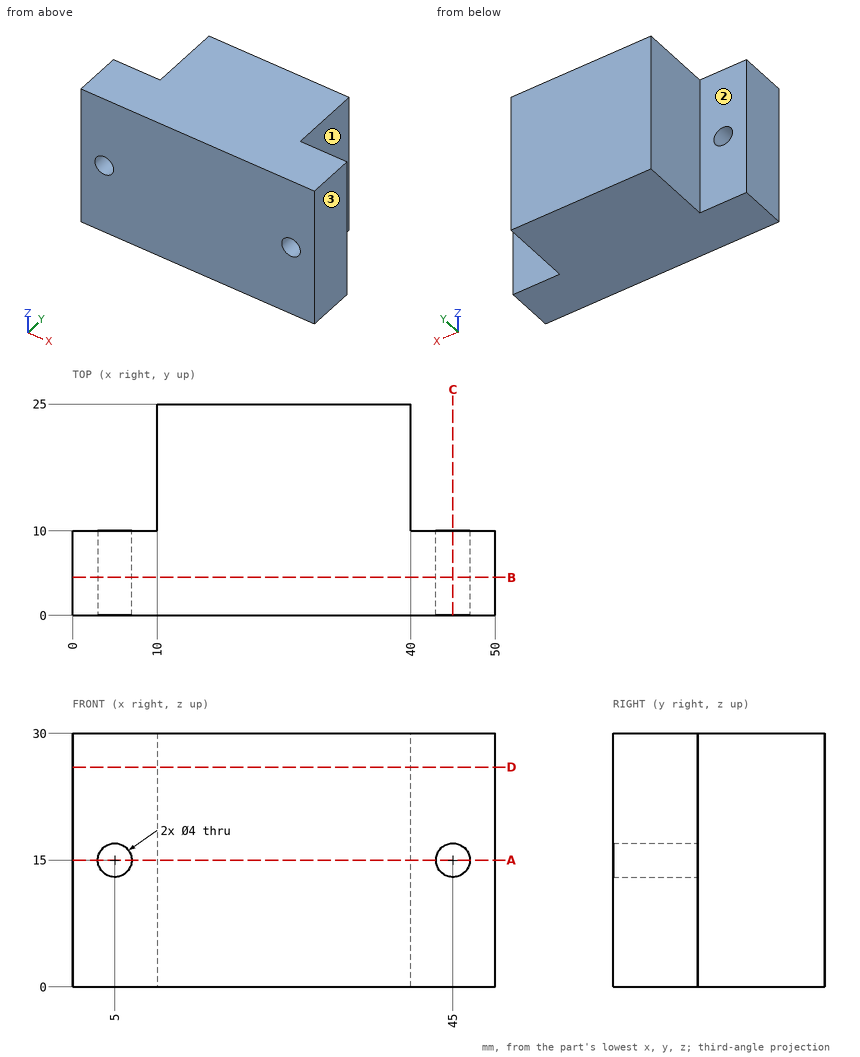
The drawing under review shows one solid part. Ordinate dimensions are in mm from its lowest x, y, z. A direction names the side the tool comes from. Round coordinates to 2 decimals unless told otherwise and drop trailing zeros. Loops run counter-clockwise (first coordinate to the right, second up) from the corner with the lowest first, then second, coordinate; pieces in that order, holes last. Notation, with made-up numbers: (43.25, 66.25) -> (53.25, 66.25) arc R22 cw to (53.25, 104.25) -> close; hole circle Ø8 at (-25, -10). An arc over 180 degrees is marked (long way). Answer in a Markdown table with one row per item.
1) Consider section B-B, the plane y = 4.5. Write out the cut boundary in (x, z), plus the area to 3 significant figures.
Taken from the geometry:
| item | result |
|---|---|
| outline | (0, 0) -> (50, 0) -> (50, 30) -> (0, 30) -> close; hole circle Ø4 at (5, 15); hole circle Ø4 at (45, 15) |
| area | 1,470 mm² |
2) Consider section A-A, the plane z = 15. Write out the cut boundary in (x, y), plus the area to 3 significant figures.
Taken from the geometry:
| item | result |
|---|---|
| outline | (0, 0) -> (3, 0) -> (3, 10) -> (0, 10) -> close; (7, 0) -> (43, 0) -> (43, 10) -> (40, 10) -> (40, 25) -> (10, 25) -> (10, 10) -> (7, 10) -> close; (47, 0) -> (50, 0) -> (50, 10) -> (47, 10) -> close |
| area | 870 mm² |
3) Tool access review of the marked faces 1, 2 and 3: name each direction out of +Z, -Z, +X, -X, +Y, -Y from which nothing blocks a thin tool from reaching the whole face with its end or side.
Taken from the geometry:
| item | result |
|---|---|
| face 1 | +Z, -Z, +X, +Y |
| face 2 | +Z, -Z, -X, +Y |
| face 3 | +Z, -Z, +X, +Y, -Y |
4) Consider section C-C, the plane x = 45. Write out the cut boundary in (y, z), plus the area to 3 significant figures.
Taken from the geometry:
| item | result |
|---|---|
| outline | (0, 0) -> (10, 0) -> (10, 13) -> (0, 13) -> close; (0, 17) -> (10, 17) -> (10, 30) -> (0, 30) -> close |
| area | 260 mm² |
5) Wall thickness on line 1 along Z through (x, y) = (5, 2); line 2 along X through (y, z) = (9.25, 14); line 3 along Y through (x, z) = (44.5, 7): over which ranges is each line inside the solid? List them lowest first.
Taken from the geometry:
| item | result |
|---|---|
| line 1 | z = 0 to 13, 17 to 30 |
| line 2 | x = 0 to 3.27, 6.73 to 43.27, 46.73 to 50 |
| line 3 | y = 0 to 10 |
6) For pin 1 Ø2 at (y, z) = (21.5, 4.5) entering from -X; pin 2 Ø4 at (x, z) = (42, 4) entering from -Y; pin 3 Ø2.5 at (x, z) = (45, 15) entering from +Y; pin 4 Ø4.5 at (y, z) = (16, 13.5) entering from +X, all flat-tipped, find the tip position at first contact; note any pin that passes through.
Taken from the geometry:
| item | result |
|---|---|
| pin 1 | stops at x = 10 |
| pin 2 | stops at y = 0 |
| pin 3 | passes through |
| pin 4 | stops at x = 40 |
7) Consider section D-D, the plane z = 26. Write out the cut boundary in (x, y), plus the area to 3 significant figures.
Taken from the geometry:
| item | result |
|---|---|
| outline | (0, 0) -> (50, 0) -> (50, 10) -> (40, 10) -> (40, 25) -> (10, 25) -> (10, 10) -> (0, 10) -> close |
| area | 950 mm² |
